Verification items for this drawing (mm, ordinates from the low corner). Coordinates: 2 decimals unless noted, no trailing zeros. Write each loop counter-clockwise with the first axis right and the second up, starting at its lowest first coordinate (ties: lowest second). Pieces come first, ordered by that corner, then holes. Notation, with made-up numbers: (-24, 34.5) -> (16, 34.5) arc R36 cw to (16, 72.5) -> close; hole circle Ø2 at (18.25, 6). An arc over 180 degrees is marked (long way). Answer as CSV lines item,"result".
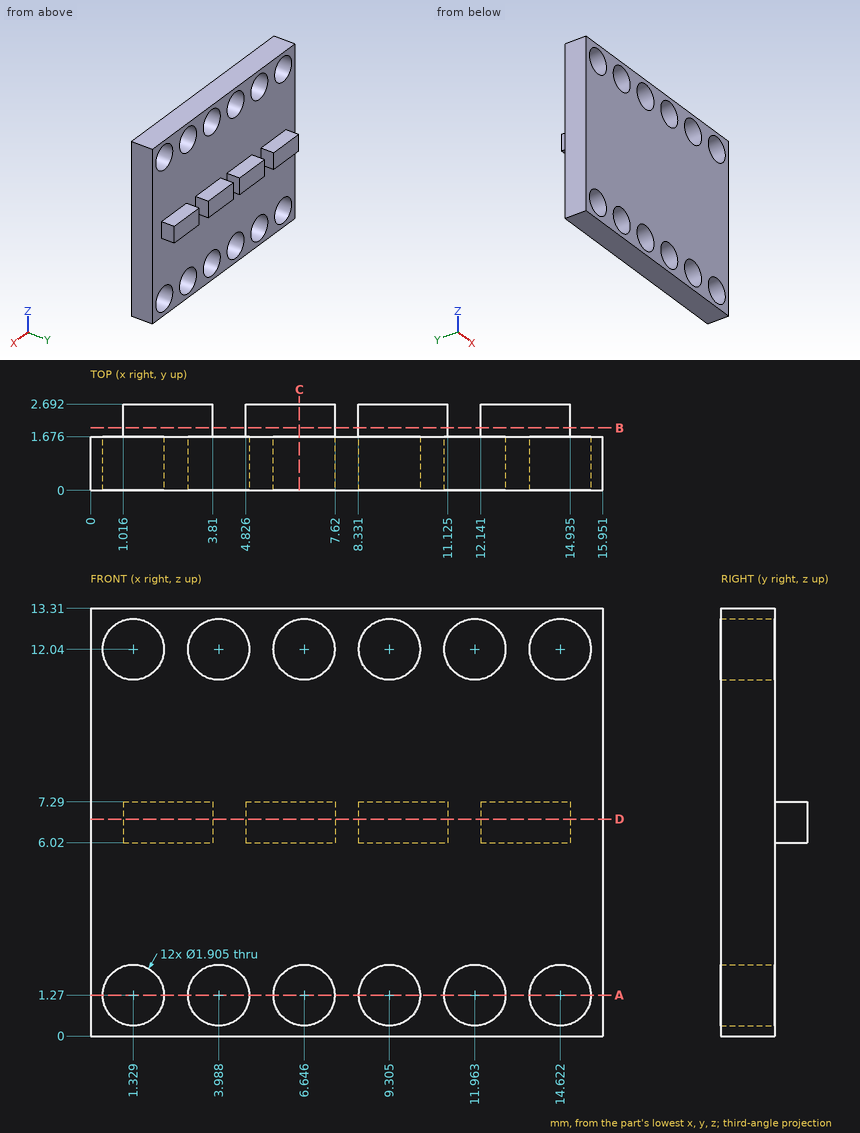
Item 1: Thickness scan on probe 1 along Z at (x, y) = (9.5, 0.3); probe 2 along Z at (x, y) = (12.5, 0.6) (1 decimal); probe 3 along Y at (x, z) = (1.5, 10). Record the ranges inside material, lowest first.
Responses:
probe 1,"z = 0 to 0.34, 2.2 to 11.11, 12.97 to 13.31"
probe 2,"z = 0 to 0.5, 2.1 to 11.3, 12.8 to 13.3"
probe 3,"y = 0 to 1.68"
Item 2: Cross-section at B-B, the plane y = 1.95. Record the cut outline in (x, z) (1 decimal).
Responses:
outline,"(1, 6) -> (3.8, 6) -> (3.8, 7.3) -> (1, 7.3) -> close; (4.8, 6) -> (7.6, 6) -> (7.6, 7.3) -> (4.8, 7.3) -> close; (8.3, 6) -> (11.1, 6) -> (11.1, 7.3) -> (8.3, 7.3) -> close; (12.1, 6) -> (14.9, 6) -> (14.9, 7.3) -> (12.1, 7.3) -> close"
Item 3: Cross-section at D-D, the plane z = 6.75. Record the cut outline in (x, y) (1 decimal).
Responses:
outline,"(0, 0) -> (16, 0) -> (16, 1.7) -> (14.9, 1.7) -> (14.9, 2.7) -> (12.1, 2.7) -> (12.1, 1.7) -> (11.1, 1.7) -> (11.1, 2.7) -> (8.3, 2.7) -> (8.3, 1.7) -> (7.6, 1.7) -> (7.6, 2.7) -> (4.8, 2.7) -> (4.8, 1.7) -> (3.8, 1.7) -> (3.8, 2.7) -> (1, 2.7) -> (1, 1.7) -> (0, 1.7) -> close"
Item 4: Cross-section at A-A, the plane z = 1.27. Count the separate pieces of the cut face and the enclosed holes in it.
Responses:
separate pieces,"7"
enclosed holes,"0"
Item 5: Depth check by flat-ended pin: pin 1 Ø1.5 at (x, z) = (9.3, 1.27) entering from +Y; pin 2 Ø1.1 at (x, y) = (13.5, 2.5) entering from +Z; pin 3 Ø1.1 at (y, z) = (2.5, 7) entering from -X. Enter the tip coordinate at first touch or a pass-through.
Responses:
pin 1,"passes through"
pin 2,"stops at z = 7.29"
pin 3,"stops at x = 1.02"
Item 6: Cross-section at C-C, the plane x = 6.5. Record the cut outline in (y, z), plus the area to 3 significant figures.
Responses:
outline,"(0, 0) -> (1.68, 0) -> (1.68, 0.33) -> (0, 0.33) -> close; (0, 2.21) -> (1.68, 2.21) -> (1.68, 6.02) -> (2.69, 6.02) -> (2.69, 7.29) -> (1.68, 7.29) -> (1.68, 11.1) -> (0, 11.1) -> close; (0, 12.98) -> (1.68, 12.98) -> (1.68, 13.31) -> (0, 13.31) -> close"
area,"17.3 mm2"
